from build123d import *

# Parameters (mm, degrees)
F2_SIZE  = 0.79375
F4_DEPTH = 12.7


with BuildPart() as f1:
    # F0 (on Front) → F1 (revolve)
    with BuildSketch(Plane.XZ):
        Polygon((7.9375, 0), (5.800725, 0), (5.800725, -50.8), (5.1, -51.221038), (5.1, -70.271038), (7.9375, -70.271038), align=None)
    revolve(axis=Axis((0, 0, -3.067858), (0, 0, -1)))

    # F2
    f2_edges = [f1.edges().sort_by_distance(p)[0] for p in [
        (-7.9375, 0, 0),
        (-7.9375, 0, -70.271038),
    ]]
    chamfer(f2_edges, length=F2_SIZE)

    # F3 (on Right) → F4 (cut, symmetric)
    with BuildSketch(Plane.YZ):
        with BuildLine():
            ThreePointArc((-4.7625, -51.221038), (0, -55.983538), (4.7625, -51.221038))
            Line((4.7625, -51.221038), (4.7625, -19.05))
            ThreePointArc((4.7625, -19.05), (0, -14.2875), (-4.7625, -19.05))
            Line((-4.7625, -19.05), (-4.7625, -51.221038))
        make_face()
    extrude(amount=F4_DEPTH, both=True, mode=Mode.SUBTRACT)


solid = f1.part
The model under review builds one solid part; all positions refer to its coordinate system, in mm. A direction names the side the tool comes from. Coordinates: 2 decimals unless noted, no trailing zeros. Write each loop counter-clockwise with the first axis right and the second up, starting at its lowest first coordinate (ties: lowest second). Pieces come first, ordered by that corner, then holes. Notation, with made-up numbers: M -25,5.25 L 18,5.25 A17 ccw 18,18.25 Z; hole C 51.25,80 d7. An arc over 180 degrees is marked long. Put each result on its own line as item: value.
1) For faces 4 (the cylindrical face through (-3.8, -3.4, -63)), 5 (the flat face through (5, -4.762, -35)), 6 (the cylindrical face through (2.677, 5.146, -20.111)), list the 3-axis set-ups (+Z, -Z, +X, -X, +Y, -Y) from which the entire face can be reached by the end or side of a thin tool; tool diameter is ignored.
Computed:
face 4: +Z, -Z
face 5: +X, -X
face 6: +Z
2) Draft analysis for pull direction Y (two halves, no side actions). For faces 1 (the cylindrical face through (-5.85, -5.365, -34.655)), 2 (the flat face through (5, 4.762, -35)), 3 (the flat face through (0, -6, 0)), state which applies: released by +Y, released by -Y, zero draft, split by the parting line, or undercut.
Computed:
face 1: split by the parting line
face 2: undercut
face 3: zero draft
3) Add section B-B on x = 0. Give the boundary of the cut face in (y, z).
Computed:
outline: M -7.94,-69.48 L -7.14,-70.27 L -5.1,-70.27 L -5.1,-51.22 L -5.8,-50.8 L -5.8,0 L -7.14,0 L -7.94,-0.79 Z; M 5.1,-70.27 L 7.14,-70.27 L 7.94,-69.48 L 7.94,-0.79 L 7.14,0 L 5.8,0 L 5.8,-50.8 L 5.1,-51.22 Z
4) Add section A-A on y = 0. Give the boundary of the cut face in (x, z).
Computed:
outline: M -7.94,-69.48 L -7.14,-70.27 L -5.1,-70.27 L -5.1,-55.98 L -7.94,-55.98 Z; M -7.94,-14.29 L -5.8,-14.29 L -5.8,0 L -7.14,0 L -7.94,-0.79 Z; M 5.1,-70.27 L 7.14,-70.27 L 7.94,-69.48 L 7.94,-55.98 L 5.1,-55.98 Z; M 5.8,-14.29 L 7.94,-14.29 L 7.94,-0.79 L 7.14,0 L 5.8,0 Z
5) Clearance check with flat-ended pins moving along their axes: pin 1 Ø5 at (x, z) = (-5, -33.5) entering from -Y; pin 2 Ø3.5 at (x, z) = (-4, -29) entering from +Y; pin 3 Ø3.5 at (x, z) = (3.5, -40) entering from +Y; pin 4 Ø9 at (x, y) = (0, 0) entering from -Z. State where each tip first meets the part, or that it passes through.
Computed:
pin 1: stops at y = -7.53
pin 2: stops at y = 7.61
pin 3: stops at y = 7.74
pin 4: passes through
6) Add section D-D on y = 3.25. State how many separate pieces and enclosed holes the cut face has, then the cut area to 3 significant figures.
Computed:
separate pieces: 4
enclosed holes: 0
area: 178 mm2
7) Wall thickness on probe 1 along Y at (x, z) = (0, -61.25); probe 2 along X at (y, z) = (0, -14): over which ranges is each line inside the solid? List them lowest first. Write a range as [from, to].
Computed:
probe 1: y = [-7.94, -5.1], [5.1, 7.94]
probe 2: x = [-7.94, -5.8], [5.8, 7.94]
